CAD build for the part. Positions are in the model's coordinates, mm. Face numbers are marked on the shaded views. A direction names the side the tool comes from. Give positions to 0.01 mm unless a question says otherwise; leave off trailing zeros. Loops run counter-clockwise (first coordinate to the right, second up) from the corner with the lowest first, then second, coordinate; pieces in that order, holes last. Notation, with made-up numbers: (19.5, 51) -> (64.5, 51) arc R31 cw to (64.5, 78) -> close; hole circle Ø4 at (-11, 72). An arc over 180 degrees is marked (long way). Use one line per item in the form item = value.
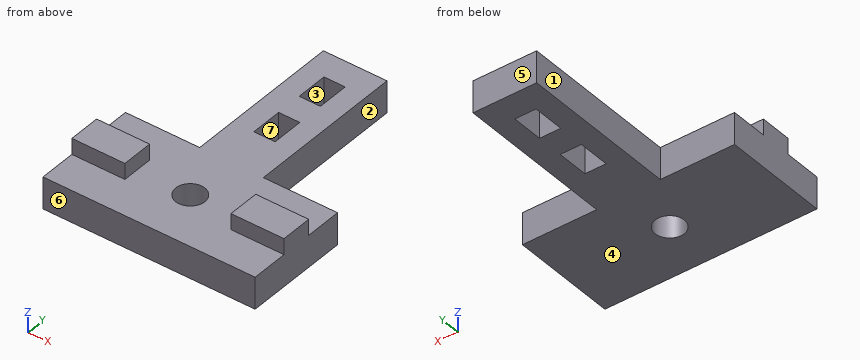
```python
from build123d import *

# Parameters (mm, degrees)
SKETCH_R     = 2.75
SKETCH_W     = 4
SKETCH_H     = 6
PAD_DEPTH    = 6
SKETCH001_W  = 10
SKETCH001_H  = 6
PAD001_DEPTH = 3


with BuildPart() as part:
    # Sketch → Pad (new body)
    with BuildSketch(Plane.XY):
        Polygon((-6, 50), (-6, 20), (-20, 20), (-20, 0), (20, 0), (20, 20), (6, 20), (6, 50), align=None)
        with Locations((0, 10)):
            Circle(SKETCH_R, mode=Mode.SUBTRACT)
        with Locations((0, 42)):
            Rectangle(SKETCH_W, SKETCH_H, mode=Mode.SUBTRACT)
        with Locations((0, 31)):
            Rectangle(SKETCH_W, SKETCH_H, mode=Mode.SUBTRACT)
    extrude(amount=PAD_DEPTH)

    # Sketch001 (on Face19 of Pad) → Pad001 (join)
    with BuildSketch(Plane.XY.offset(6)):
        with Locations((-15, 10)):
            Rectangle(SKETCH001_W, SKETCH001_H)
        with Locations((15, 10)):
            Rectangle(SKETCH001_W, SKETCH001_H)
    extrude(amount=PAD001_DEPTH)


solid = part.part
```
1. Cut at B-B, the plane y = 44. Write the cut outline in (x, z), then the cut area to 3 significant figures.
Result sheet:
outline = (-6, 0) -> (-2, 0) -> (-2, 6) -> (-6, 6) -> close; (2, 0) -> (6, 0) -> (6, 6) -> (2, 6) -> close
area = 48.0 mm^2
2. Mould opens along Y. For the marked faces 5, 6 and 7 say: pulls with the +Y half, pulls with the -Y half, needs draft (parallel to the pull), parting line crosses it, or undercut.
Result sheet:
face_5 = pulls with the +Y half
face_6 = pulls with the -Y half
face_7 = undercut
3. Drill centre lines: line 1 (Y direction, x = 0, z = 4.55); line 2 (Z direction, x = 3, y = 27.5); line 3 (Y direction, x = 1, z = 3.75). Where is each one in solid material? Low to high.
Result sheet:
line_1 = 0 to 7.25, 12.75 to 28, 34 to 39, 45 to 50
line_2 = 0 to 6
line_3 = 0 to 7.44, 12.56 to 28, 34 to 39, 45 to 50
4. Cut at C-C, the plane z = 7.75. Write the cut outline in (x, y), then the cut area to 3 significant figures.
Result sheet:
outline = (-20, 7) -> (-10, 7) -> (-10, 13) -> (-20, 13) -> close; (10, 7) -> (20, 7) -> (20, 13) -> (10, 13) -> close
area = 120 mm^2
5. Tool access for the marked faces 1, 2, 3 and 4: list every direction of +Z, -Z, +X, -X, +Y, -Y with a clear straight run to the whole face (end or side of a thin tool).
Result sheet:
face_1 = +Z, -Z, -X, +Y
face_2 = +Z, -Z, +X, +Y
face_3 = +Z, -Z
face_4 = -Z, +X, -X, +Y, -Y
6. Cut at A-A, the plane x = 0. Write the cut outline in (y, z).
Result sheet:
outline = (0, 0) -> (7.25, 0) -> (7.25, 6) -> (0, 6) -> close; (12.75, 0) -> (28, 0) -> (28, 6) -> (12.75, 6) -> close; (34, 0) -> (39, 0) -> (39, 6) -> (34, 6) -> close; (45, 0) -> (50, 0) -> (50, 6) -> (45, 6) -> close
7. Cut at D-D, the plane z = 1. Write the cut outline in (x, y), then the cut area to 3 significant figures.
Result sheet:
outline = (-20, 0) -> (20, 0) -> (20, 20) -> (6, 20) -> (6, 50) -> (-6, 50) -> (-6, 20) -> (-20, 20) -> close; hole circle Ø5.5 at (0, 10); hole (-2, 28) -> (2, 28) -> (2, 34) -> (-2, 34) -> close; hole (-2, 39) -> (2, 39) -> (2, 45) -> (-2, 45) -> close
area = 1,090 mm^2
8. Drop flat-ended pins along their axis: P1, Ø3.5, axis at x = 17.5, z = 7.5, coming from the +Y side; P2, Ø1.8, axis at y = 32, z = 2, coming from the +X side; P3, Ø3, axis at y = 32.5, z = 4, coming from the -X side; P4, Ø10, axis at x = 14, y = 36.5, coming from the -Z side. Give the stop position or say it passes through.
Result sheet:
P1 = 20
P2 = 6
P3 = -6
P4 = through
